The figure shows three views and two pictorial views of one solid part (mm, origin at its lowest corner). Answer the questions. A direction names the side the tool comes from. Give positions to 0.01 mm unless a question says otherwise; leave off trailing zeros. Loops run counter-clockwise (first coordinate to the right, second up) from the corner with the lowest first, then second, coordinate; pieces in that order, holes last.
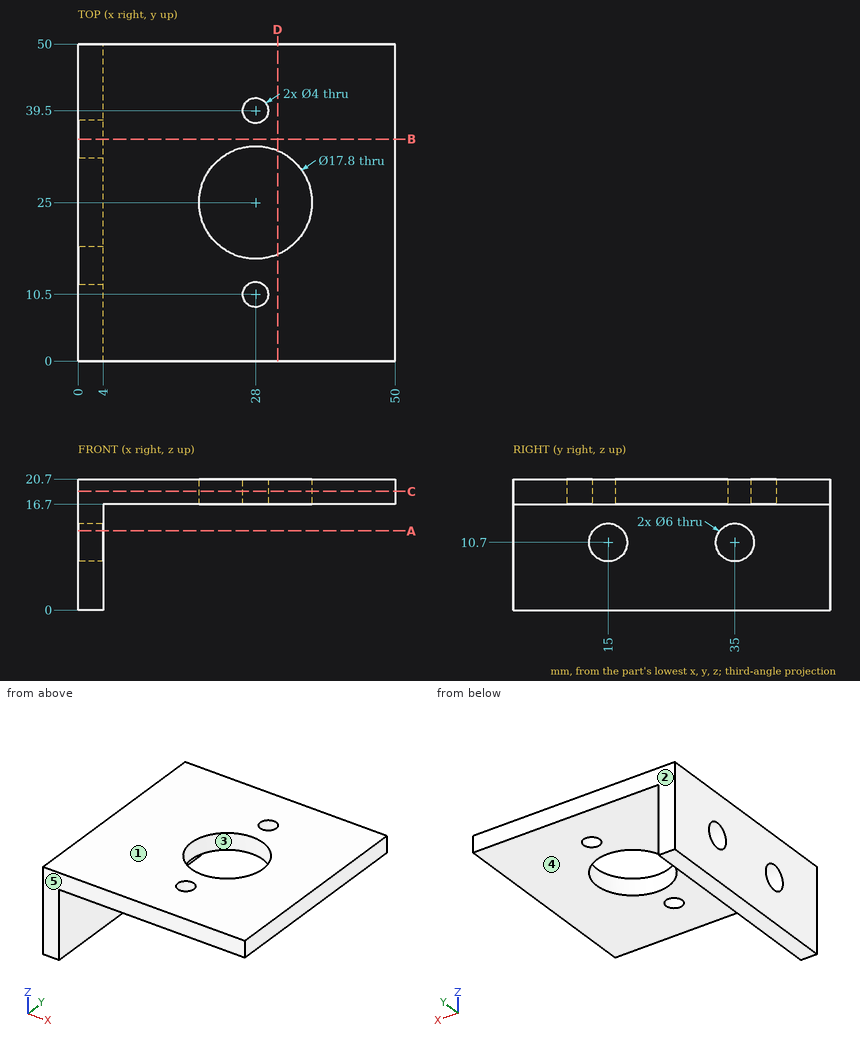
Q1. Determine the mould class of the marked faces 1, 2 and 3 for opening direction Y: +Y half, -Y half, draft (parallel to the pull), parting line (faces both ways), or undercut.
Q2. Section C-C on z = 18.75 is taken. Give the vertices of the cut face in (x, y), plus the area to 3 significant figures.
Q3. Section D-D on x = 31.5 is taken. Give the vertices of the cut face in (y, z), plus the area to 3 significant figures.
Q4. Given pin 1 (2 mm diameter, centred on x = 6, y = 34.5, fed in from -Z); pin 2 (7 mm diameter, centred on y = 35, z = 10.7, fed in from +X), each flat-ended and moving along its own axis, determine where each tip first touches the part or whether it passes through.
Q5. Which of the six approach directions +Z, -Z, +X, -X, +Y, -Y give full straight-line access (tool end or side, diameter ignored) to the marked faces 4 and 5?
Q6. Section A-A on z = 12.5 is taken. Give the vertices of the cut face in (x, y).
Q7. Section B-B on y = 35 is taken. Give the vertices of the cut face in (x, z), plus the area to 3 significant figures.
Q8. Consider line 1 along Y through (x, z) = (2.7, 10.7); line 2 along Y through (x, z) = (28, 19.2); line 3 along X through (y, z) = (27, 12). Determine where each line is inside the solid, lowest interval first.
Check result:
1. face 1: draft
1. face 2: +Y half
1. face 3: undercut
2. outline: (0, 0) - (50, 0) - (50, 50) - (0, 50) - close; hole circle Ø17.8 at (28, 25); hole circle Ø4 at (28, 10.5); hole circle Ø4 at (28, 39.5)
2. area: 2,230 mm2
3. outline: (0, 16.7) - (16.82, 16.7) - (16.82, 20.7) - (0, 20.7) - close; (33.18, 16.7) - (50, 16.7) - (50, 20.7) - (33.18, 20.7) - close
3. area: 135 mm2
4. pin 1: stops at z = 16.7
4. pin 2: stops at x = 4
5. face 4: -Z, +X, +Y, -Y
5. face 5: +Z, -Z, +X, -X, -Y
6. outline: (0, 0) - (4, 0) - (4, 12.6) - (0, 12.6) - close; (0, 17.4) - (4, 17.4) - (4, 32.6) - (0, 32.6) - close; (0, 37.4) - (4, 37.4) - (4, 50) - (0, 50) - close
7. outline: (0, 0) - (4, 0) - (4, 7.7) - (0, 7.7) - close; (0, 13.7) - (4, 13.7) - (4, 16.7) - (50, 16.7) - (50, 20.7) - (0, 20.7) - close
7. area: 243 mm2
8. line 1: y = 0 to 12, 18 to 32, 38 to 50
8. line 2: y = 0 to 8.5, 12.5 to 16.1, 33.9 to 37.5, 41.5 to 50
8. line 3: x = 0 to 4
